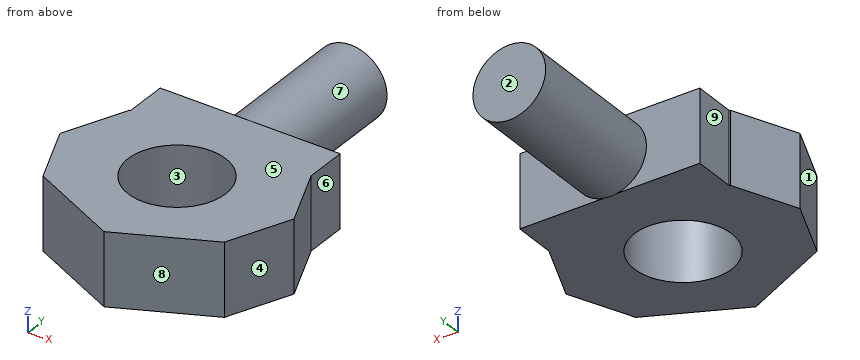
```python
from build123d import *

# Parameters (mm, degrees)
SKETCH1_R           = 6.694456565
BOSS_EXTRUDE1_DEPTH = 10
SKETCH2_W           = 24.765512155
SKETCH2_H           = 10
BOSS_EXTRUDE2_DEPTH = 7
SKETCH4_R           = 5
BOSS_EXTRUDE4_DEPTH = 20


with BuildPart() as part:
    # Sketch1 → Boss-Extrude1 (new body)
    with BuildSketch(Plane.XY):
        Polygon((-12.471629347, -23.064398423), (-16.102258105, -14.474005392), (-12.471629347, -5.883612362), (0, 0), (12.471629347, -5.883612362), (16.102258105, -14.474005392), (12.471629347, -23.064398423), (0, -28.948010785), align=None)
        with Locations((0, -14.474005392)):
            Circle(SKETCH1_R, mode=Mode.SUBTRACT)
    extrude(amount=BOSS_EXTRUDE1_DEPTH)

    # Sketch2 → Boss-Extrude2 (add)
    with BuildSketch(Plane(origin=(0, 0, 0), x_dir=(1, 0, 0), z_dir=(0, 1, 0))):
        with Locations((0.039254209, -5)):
            Rectangle(SKETCH2_W, SKETCH2_H)
    extrude(amount=-BOSS_EXTRUDE2_DEPTH)

    # Sketch4 → Boss-Extrude4 (add)
    with BuildSketch(Plane(origin=(0, 0, 0), x_dir=(1, 0, 0), z_dir=(0, 1, 0))):
        with Locations(Location((0, -4.912660405, 0), (0, 0, 100.724879792))):
            Circle(SKETCH4_R)
    extrude(amount=BOSS_EXTRUDE4_DEPTH)


solid = part.part
```
Can you work these out from the model? Positions are in its coordinate system, mm. Face numbers are marked on the shaded views. A direction names the side the tool comes from. Coordinates: 2 decimals unless noted, no trailing zeros. Order: outer loops, then holes, each group sorted by start corner. A loop starts at its lowest first (then second) coordinate and runs counter-clockwise, first axis right, second up.
1. If we section it at C-C (y = -8.5): Please give me the cut outline in (x, z).
2. I'm going to push flat-ended pins straight in: pin 1 (2 mm diameter, centred on y = 5, z = 2, fed in from +X); pin 2 (3 mm diameter, centred on y = -4, z = 3.5, fed in from +X); pin 3 (2 mm diameter, centred on y = -19, z = 5, fed in from +X); pin 4 (6 mm diameter, centred on x = -7, z = 8.5, fed in from +Y). Where does each tip first touch, or does it pass through?
3. Thinking about a two-plate mould opening in X: for the marked faces 1, 2, 3 and 4, which applies, +X half, -X half, draft (parallel to the pull), parting line (faces both ways), or undercut?
4. If we section it at D-D (y = 1): Please give me the cut outline in (x, z), then the cut area to 3 significant figures.
5. I need wall thicknesses on line 1 (Y direction, x = 0, z = 5); line 2 (Z direction, x = -6, y = -18.5); line 3 (Y direction, x = 5, z = 0.75). Which ranges of each line are inside material? Lowest first, please.
6. If we section it at A-A (z = 2.75): Please give me the cut outline in (x, y).
7. If we section it at B-B (x = 3): Please give me the cut outline in (y, z), then the cut area to 3 significant figures.
8. For the marked faces 5, 6, 7, 8 and 9, which set-ups out of +Z, -Z, +X, -X, +Y, -Y let a thin tool reach every point of the face, with its end or its side?
Entries:
1. outline: (-13.58, 0) - (-3.02, 0) - (-3.02, 10) - (-13.58, 10) - close; (3.02, 0) - (13.58, 0) - (13.58, 10) - (3.02, 10) - close
2. pin 1: stops at x = 4.62
2. pin 2: stops at x = 12.42
2. pin 3: stops at x = 14.61
2. pin 4: stops at y = 20
3. face 1: -X half
3. face 2: draft
3. face 3: undercut
3. face 4: +X half
4. outline: circle Ø10 at (0, 4.91)
4. area: 78.5 mm2
5. line 1: y = -28.95 to -21.17, -7.78 to 20
5. line 2: z = 0 to 10
5. line 3: y = -26.59 to -18.93, -10.02 to 0
6. outline: (-16.1, -14.47) - (-12.47, -23.06) - (0, -28.95) - (12.47, -23.06) - (16.1, -14.47) - (12.47, -5.88) - (12.42, -5.86) - (12.42, 0) - (4.51, 0) - (4.51, 20) - (-4.51, 20) - (-4.51, 0) - (-12.34, 0) - (-12.34, -5.82) - (-12.47, -5.88) - close; hole circle Ø13.39 at (0, -14.47)
7. outline: (-27.53, 0) - (-20.46, 0) - (-20.46, 10) - (-27.53, 10) - close; (-8.49, 0) - (0, 0) - (0, 0.91) - (20, 0.91) - (20, 8.91) - (0, 8.91) - (0, 10) - (-8.49, 10) - close
7. area: 316 mm2
8. face 5: +Z, +X, -X, +Y, -Y
8. face 6: +Z, -Z, +X, +Y
8. face 7: +Y
8. face 8: +Z, -Z, +X, -Y
8. face 9: +Z, -Z, -X, +Y
